```python
from build123d import *

# Parameters (mm, degrees)
SKETCH1_W           = 80.2
SKETCH1_H           = 80.2
SKETCH1_R           = 2.05
BOSS_EXTRUDE1_DEPTH = 5
CHAMFER1_SIZE       = 2.3
FILLET1_R           = 5
FILLET2_R           = 1
SKETCH2_R           = 4.55
BOSS_EXTRUDE2_DEPTH = 1


with BuildPart() as part:
    # Sketch1 → Boss-Extrude1 (new body)
    with BuildSketch(Plane.XY):
        with BuildLine():
            ThreePointArc((82.7, -2.05), (85.917335854, 5.717335854), (78.15, 2.5))
            Line((78.15, 2.5), (2.05, 2.5))
            ThreePointArc((2.05, 2.5), (-5.717335854, 5.717335854), (-2.5, -2.05))
            Line((-2.5, -2.05), (-2.5, -78.15))
            ThreePointArc((-2.5, -78.15), (-5.717335854, -85.917335854), (2.05, -82.7))
            Line((2.05, -82.7), (78.15, -82.7))
            ThreePointArc((78.15, -82.7), (85.917335854, -85.917335854), (82.7, -78.15))
            Line((82.7, -78.15), (82.7, -2.05))
        make_face()
        with Locations((40.1, -40.1)):
            Rectangle(SKETCH1_W, SKETCH1_H, mode=Mode.SUBTRACT)
        with Locations((82.7, -82.7)):
            Circle(SKETCH1_R, mode=Mode.SUBTRACT)
        with Locations((-2.5, -82.7)):
            Circle(SKETCH1_R, mode=Mode.SUBTRACT)
        with Locations((82.7, 2.5)):
            Circle(SKETCH1_R, mode=Mode.SUBTRACT)
        with Locations((-2.5, 2.5)):
            Circle(SKETCH1_R, mode=Mode.SUBTRACT)
    extrude(amount=BOSS_EXTRUDE1_DEPTH)

    # Chamfer1
    chamfer1_edges = [part.edges().sort_by_distance(p)[0] for p in [
        (0, 0, 2.5),
        (0, -80.2, 2.5),
        (80.2, -80.2, 2.5),
        (80.2, 0, 2.5),
    ]]
    chamfer(chamfer1_edges, length=CHAMFER1_SIZE)

    # Fillet1
    fillet1_edges = [part.edges().sort_by_distance(p)[0] for p in [
        (2.05, 2.5, 2.5),
        (78.15, 2.5, 2.5),
        (82.7, -2.05, 2.5),
        (82.7, -78.15, 2.5),
        (78.15, -82.7, 2.5),
        (2.05, -82.7, 2.5),
        (-2.5, -78.15, 2.5),
        (-2.5, -2.05, 2.5),
    ]]
    fillet(fillet1_edges, radius=FILLET1_R)

    # Fillet2
    fillet2_edges = [part.edges().sort_by_distance(p)[0] for p in [
        (80.65, 2.5, 5),
        (80.65, -82.7, 5),
        (-4.55, 2.5, 5),
        (-4.55, -82.7, 5),
    ]]
    fillet(fillet2_edges, radius=FILLET2_R)

    # Sketch2 → Boss-Extrude2 (add)
    with BuildSketch(Plane(origin=(0, 0, 0), x_dir=(-1, 0, 0), z_dir=(0, 0, -1))):
        with Locations((-82.7, 2.5)):
            Circle(SKETCH2_R)
        with Locations((2.5, 2.5)):
            Circle(SKETCH2_R)
        with Locations((2.5, -82.7)):
            Circle(SKETCH2_R)
        with Locations((-82.7, -82.7)):
            Circle(SKETCH2_R)
    extrude(amount=-BOSS_EXTRUDE2_DEPTH)


solid = part.part
```
Read the model definition and answer for the solid it produces. Units are mm, in the model's axes. A direction names the side the tool comes from. Give positions to 0.01 mm unless a question says otherwise; leave off trailing zeros. Write each loop counter-clockwise with the first axis right and the second up, starting at its lowest first coordinate (ties: lowest second). Pieces come first, ordered by that corner, then holes. Notation, with made-up numbers: M -35,-27.75 L 20,-27.75 A22 ccw 20,-15.75 Z; hole C -7,77.5 d8. An arc over 180 degrees is marked long. Put each result on its own line as item: value. Start each with the question number.
1. Each of these flat-tipped pins is pushed along its axis until it touches: pin 1 Ø1.5 at (x, z) = (46.5, 3) entering from +Y; pin 2 Ø2.5 at (x, z) = (37.5, 2) entering from -Y; pin 3 Ø5.5 at (x, y) = (-2.5, -82.7) entering from +Z. Where does it stop, or does it pass through?
2. Which of the six approach directions +Z, -Z, +X, -X, +Y, -Y give full straight-line access (tool end or side, diameter ignored) to faces 1 (the cylindrical face through (3.227, 3.119, 2.535)), 2 (the cylindrical face through (-3.15, -3.17, 2.54)), 3 (the flat face through (40, -82.7, 2)), 4 (the cylindrical face through (-2.767, -80.667, 2.479)), 5 (the flat face through (80.2, -41, 2))?
3. The part is cut by section C-C, the plane z = 1.95. Give the vertices of the cut face in (x, y).
4. The part is cut by section B-B, the plane x = 51. Give the vertices of the cut face in (y, z), and give its area (3 significant figures).
5. Consider line 1 along X through (y, z) = (-30.5, 4.3); line 2 along Y through (x, z) = (35, 4.7); line 3 along X through (y, z) = (-4.5, 3.8). Determine where each line is inside the solid, lowest interval first.
6. For a pull along Y with two mould halves and no side action, classify faces 6 (the cylindrical face through (77.03, 3.15, 2.54)), 7 (the cylindrical face through (83.35, -3.17, 2.54)), 8 (the cylindrical face through (77.03, -83.35, 2.54)) as released by +Y, released by -Y, zero draft, split by the parting line, or undercut.
7. The part is cut by section A-A, the plane y = -60.5. Give the vertices of the cut face in (x, z).
Final values:
1. pin 1: stops at y = 2.5
1. pin 2: stops at y = -82.7
1. pin 3: stops at z = 4.95
2. face 1: +Z, -Z, +Y
2. face 2: +Z, -Z, -X
2. face 3: +Z, -Z, -Y
2. face 4: +Z
2. face 5: +Z, -Z
3. outline: M -4.88,-78.82 A4.55 ccw long 1.38,-85.08 A5 cw 5.64,-82.7 L 74.56,-82.7 A5 cw 78.82,-85.08 A4.55 ccw long 85.08,-78.82 A5 cw 82.7,-74.56 L 82.7,-5.64 A5 cw 85.08,-1.38 A4.55 ccw long 78.82,4.88 A5 cw 74.56,2.5 L 5.64,2.5 A5 cw 1.38,4.88 A4.55 ccw long -4.88,-1.38 A5 cw -2.5,-5.64 L -2.5,-74.56 A5 cw Z; hole C -2.5,-82.7 d4.1; hole C -2.5,2.5 d4.1; hole M 0,-77.9 L 2.3,-80.2 L 77.9,-80.2 L 80.2,-77.9 L 80.2,-2.3 L 77.9,0 L 2.3,0 L 0,-2.3 Z; hole C 82.7,-82.7 d4.1; hole C 82.7,2.5 d4.1
4. outline: M -82.7,0 L -80.2,0 L -80.2,5 L -82.7,5 Z; M 0,0 L 2.5,0 L 2.5,5 L 0,5 Z
4. area: 25.0 mm²
5. line 1: x = -2.5 to 0, 80.2 to 82.7
5. line 2: y = -82.7 to -80.2, 0 to 2.5
5. line 3: x = -2.63 to 0, 80.2 to 82.83
6. face 6: released by +Y
6. face 7: undercut
6. face 8: released by -Y
7. outline: M -2.5,0 L 0,0 L 0,5 L -2.5,5 Z; M 80.2,0 L 82.7,0 L 82.7,5 L 80.2,5 Z
